```python
from build123d import *

# Parameters (mm, degrees)
F0_W     = 152.4
F0_H     = 76.2
F0_R     = 3.175
F0_R_2   = 3.2004
F0_R_3   = 3.3782
F0_R_4   = 3.5687
F0_R_5   = 4.7625
F0_R_6   = 4.7879
F0_R_7   = 4.826
F0_R_8   = 4.9657
F0_R_9   = 3.683
F0_R_10  = 9.652
F0_R_11  = 5.0419
F0_R_12  = 5.55625
F0_R_13  = 5.5626
F0_R_14  = 5.56895
F0_R_15  = 5.7531
F0_R_16  = 6.35
F0_R_17  = 6.4135
F0_R_18  = 6.477
F0_R_19  = 9.525
F0_R_20  = 5.842
F0_R_21  = 9.9187
F0_R_22  = 6.7437
F0_R_23  = 6.8326
F0_R_24  = 7.1374
F1_DEPTH = 6.35
F2_R     = 5.08
F3_R     = 10.16
F4_R     = 12.7
F5_R     = 19.05
F7_D     = 6.7564
F9_D     = 9.8044
F11_D    = 11.5062


with BuildPart() as f1:
    # F0 (on Front) → F1 (new body)
    with BuildSketch(Plane.XZ):
        Rectangle(F0_W, F0_H)
        with Locations((-57.2099471569, -25.400005281)):
            Circle(F0_R, mode=Mode.SUBTRACT)
        with Locations((-38.1599462152, -25.400005281)):
            Circle(F0_R_2, mode=Mode.SUBTRACT)
        with Locations((-19.1099462152, -25.400005281)):
            Circle(F0_R_3, mode=Mode.SUBTRACT)
        with Locations((-0.0599462152, -25.400005281)):
            Circle(F0_R_4, mode=Mode.SUBTRACT)
        with Locations((-57.2099471569, -12.7)):
            Circle(F0_R_5, mode=Mode.SUBTRACT)
        with Locations((-38.1599462152, -12.7)):
            Circle(F0_R_6, mode=Mode.SUBTRACT)
        with Locations((-19.1099462152, -12.7)):
            Circle(F0_R_7, mode=Mode.SUBTRACT)
        with Locations((-0.0599462152, -12.7)):
            Circle(F0_R_8, mode=Mode.SUBTRACT)
        with Locations((18.9900537848, -25.400005281)):
            Circle(F0_R_9, mode=Mode.SUBTRACT)
        with Locations((48.5375337303, -25.400005281)):
            Circle(F0_R_10, mode=Mode.SUBTRACT)
        with Locations((18.9900537848, -12.7)):
            Circle(F0_R_11, mode=Mode.SUBTRACT)
        with Locations((-57.2099462152, 12.7)):
            Circle(F0_R_12, mode=Mode.SUBTRACT)
        with Locations((-38.1599462152, 12.7)):
            Circle(F0_R_13, mode=Mode.SUBTRACT)
        with Locations((-19.1099462152, 12.7)):
            Circle(F0_R_14, mode=Mode.SUBTRACT)
        with Locations((-0.0599462152, 12.7)):
            Circle(F0_R_15, mode=Mode.SUBTRACT)
        with Locations((-48.25777933, 25.4)):
            Circle(F0_R_16, mode=Mode.SUBTRACT)
        with Locations((-27.8356466442, 25.4)):
            Circle(F0_R_17, mode=Mode.SUBTRACT)
        with Locations((-9.6515566111, 25.4)):
            Circle(F0_R_18, mode=Mode.SUBTRACT)
        with Locations((35.668797791, 0)):
            Circle(F0_R_19, mode=Mode.SUBTRACT)
        with Locations((18.9900537848, 12.7)):
            Circle(F0_R_20, mode=Mode.SUBTRACT)
        with Locations((60.0075013936, 0)):
            Circle(F0_R_21, mode=Mode.SUBTRACT)
        with Locations((9.3718003482, 25.4)):
            Circle(F0_R_22, mode=Mode.SUBTRACT)
        with Locations((31.4724631608, 25.4)):
            Circle(F0_R_23, mode=Mode.SUBTRACT)
        with Locations((54.412394762, 25.4)):
            Circle(F0_R_24, mode=Mode.SUBTRACT)
    extrude(amount=F1_DEPTH)

    # F2
    f2_edges = [f1.edges().sort_by_distance(p)[0] for p in [
        (-76.2, -3.175, 38.1),
    ]]
    fillet(f2_edges, radius=F2_R)

    # F3
    f3_edges = [f1.edges().sort_by_distance(p)[0] for p in [
        (-76.2, -3.175, -38.1),
    ]]
    fillet(f3_edges, radius=F3_R)

    # F4
    f4_edges = [f1.edges().sort_by_distance(p)[0] for p in [
        (76.2, -3.175, -38.1),
    ]]
    fillet(f4_edges, radius=F4_R)

    # F5
    f5_edges = [f1.edges().sort_by_distance(p)[0] for p in [
        (76.2, -3.175, 38.1),
    ]]
    fillet(f5_edges, radius=F5_R)

    # F7 (through all)
    with Locations(Plane.XZ.offset(6.35)):
        with Locations((-66.7602941394, 0)):
            Hole(F7_D / 2)

    # F9 (through all)
    with Locations(Plane.XZ.offset(6.35)):
        with Locations((-47.1701584756, 0)):
            Hole(F9_D / 2)

    # F11 (through all)
    with Locations(Plane.XZ.offset(6.35)):
        with Locations((-27.8289690614, 0)):
            Hole(F11_D / 2)


solid = f1.part
```
For this review, take the finished solid that the model builds, in its own axes (mm). Coordinates: 2 decimals unless noted, no trailing zeros. Write each loop counter-clockwise with the first axis right and the second up, starting at its lowest first coordinate (ties: lowest second). Pieces come first, ordered by that corner, then holes. Notation, with made-up numbers: (81.5, -10) - (118.5, -10) arc R27 ccw to (118.5, 13) - close; hole circle Ø3 at (24.5, 75.25). An arc over 180 degrees is marked (long way). Put each result on its own line as item: value.
1. For pin 1 (9 mm diameter, centred on x = 18.99, z = -12.7, fed in from -Y), flat-tipped, find the tip position at first contact; note if it passes through.
Values found:
pin 1: through
2. Add section B-B, the plane z = 12.7. Give the boundary of the cut face in (x, y), then the cut area to 3 significant figures.
Values found:
outline: (-76.2, -6.35) - (-62.77, -6.35) - (-62.77, 0) - (-76.2, 0) - close; (-51.65, -6.35) - (-43.72, -6.35) - (-43.72, 0) - (-51.65, 0) - close; (-32.6, -6.35) - (-24.68, -6.35) - (-24.68, 0) - (-32.6, 0) - close; (-13.54, -6.35) - (-5.81, -6.35) - (-5.81, 0) - (-13.54, 0) - close; (5.69, -6.35) - (13.15, -6.35) - (13.15, 0) - (5.69, 0) - close; (24.83, -6.35) - (76.2, -6.35) - (76.2, 0) - (24.83, 0) - close
area: 609 mm²
3. Wall thickness on probe 1 along Z at (x, y) = (29, -3); probe 2 along Z at (x, y) = (60, -3.75); probe 3 along Z at (x, y) = (1.5, -3): over which ranges is each line inside the solid? List them lowest first.
Values found:
probe 1: -38.1 to -6.8, 6.8 to 19.03, 31.77 to 38.1
probe 2: -38.1 to -9.92, 9.92 to 20.96, 29.84 to 37.89
probe 3: -38.1 to -28.61, -22.19 to -17.41, -7.99 to 7.16, 18.24 to 38.1
4. Add section A-A, the plane z = 0. Give the boundary of the cut face in (x, y), then the cut area to 3 significant figures.
Values found:
outline: (-76.2, -6.35) - (-70.14, -6.35) - (-70.14, 0) - (-76.2, 0) - close; (-63.38, -6.35) - (-52.07, -6.35) - (-52.07, 0) - (-63.38, 0) - close; (-42.27, -6.35) - (-33.58, -6.35) - (-33.58, 0) - (-42.27, 0) - close; (-22.08, -6.35) - (26.14, -6.35) - (26.14, 0) - (-22.08, 0) - close; (45.19, -6.35) - (50.09, -6.35) - (50.09, 0) - (45.19, 0) - close; (69.93, -6.35) - (76.2, -6.35) - (76.2, 0) - (69.93, 0) - close
area: 543 mm²
5. Mouldability with a two-part tool opening along X and no side actions: class faces 1 (the flat face through (-2, -3, -38.1)), 2 (the cylindrical face through (-42.273, -3.131, 0.216)), 3 (the flat face through (-76.2, -3, 2)) as released by +X, released by -X, zero draft, split by the parting line, or undercut.
Values found:
face 1: zero draft
face 2: undercut
face 3: released by -X
6. Add section C-C, the plane y = -1. Count the separate pieces of the cut face and the enclosed holes in it, then the cut area to 3 significant figures.
Values found:
separate pieces: 1
enclosed holes: 27
area: 8,470 mm²
